For this review, take the finished solid that the model builds, in its own axes (mm). Face numbers are marked on the shaded views. Coordinates: 2 decimals unless noted, no trailing zeros. Order: outer loops, then holes, each group sorted by start corner. A loop starts at its lowest first (then second) coordinate and runs counter-clockwise, first axis right, second up. Notation, with made-up numbers: (61.25, 10.5) -> (91.25, 10.5) arc R22 cw to (91.25, 33.5) -> close; hole circle Ø5 at (20, -26). An arc over 180 degrees is marked (long way). Return JSON: item names as keys, results as strings. Group by question number.
Item 1: Take a section at B-B (z = -2.3). Write out the cut boundary in (x, y).
Item 2: Draft analysis for pull direction Z (two halves, no side actions). For the marked faces 1, 2 and 3, state which applies: +Z half, -Z half, draft (parallel to the pull), parting line (faces both ways), or undercut.
Item 3: Insertion check: pin 1 (0.5 mm diameter, centred on x = 4, y = 4.5, fed in from +Z); pin 2 (1.5 mm diameter, centred on x = 0.5, z = -2, fed in from +Y); pin 3 (0.5 mm diameter, centred on y = -0.5, z = -1.5, fed in from +X). Each pin has a flat end and moves straight along its axis. Give the tip position at first contact, or say it passes through.
Item 4: Take a section at A-A (y = 6.25). Write out the cut boundary in (x, z).
Item 5: Take a section at C-C (x = 4.45). Write out the cut boundary in (y, z), then the cut area to 3 significant figures.
Item 6: Take a section at D-D (y = 1.25). Write out the cut boundary in (x, z).
Item 7: For line 1 along X through (y, z) = (-1.25, -1.1); line 2 along Y through (x, z) = (3, -1.85); line 3 along Z through (x, y) = (1.5, 7), list the stretches that pass through material, from the lowest coordinate up.
```python
from build123d import *
from OCP.BRepFilletAPI import BRepFilletAPI_MakeChamfer

# Parameters (mm, degrees)
BOSS_EXTRUDE1_DEPTH         = 2.5
SKETCH2_W                   = 5.04
SKETCH2_H                   = 1.5
CUT_EXTRUDE1_DEPTH          = 0.5
SKETCH4_W                   = 0.04
SKETCH4_H                   = 1.8
CUT_EXTRUDE2_DEPTH          = 0.04
BOSS_EXTRUDE2_START         = -5.5
SKETCH3_W                   = 0.64
SKETCH3_H                   = 0.64
BOSS_EXTRUDE2_DEPTH         = 11.5
CHAMFER1_SIZE               = 0.2
CHAMFER1_SIZE2              = 0.140041508
LPATTERN1_COUNT             = 2
LPATTERN1_PITCH             = 2.54
CHAMFER1_OF_LPATTERN1_SIZE  = 0.2
CHAMFER1_OF_LPATTERN1_SIZE2 = 0.140041508


with BuildPart() as part:
    # Sketch1 → Boss-Extrude1 (new body)
    with BuildSketch(Plane(origin=(0, 0, 0), x_dir=(1, 0, 0), z_dir=(0, 1, 0))):
        Polygon((0, 2.15), (0.35, 2.5), (2.15, 2.5), (2.5, 2.15), (2.54, 2.15), (2.89, 2.5), (4.69, 2.5), (5.04, 2.15), (5.04, 0.35), (4.69, 0), (2.89, 0), (2.54, 0.35), (2.5, 0.35), (2.15, 0), (0.35, 0), (0, 0.35), align=None)
    extrude(amount=BOSS_EXTRUDE1_DEPTH)

    # Sketch2 → Cut-Extrude1 (cut)
    with BuildSketch(Plane.XZ):
        with Locations((2.52, -1.25)):
            Rectangle(SKETCH2_W, SKETCH2_H)
    extrude(amount=-CUT_EXTRUDE1_DEPTH, mode=Mode.SUBTRACT)

    # Sketch4 → Cut-Extrude2 (cut)
    with BuildSketch(Plane(origin=(0, 2.5, 0), x_dir=(1, 0, 0), z_dir=(0, 1, 0))):
        with Locations((5.06, 1.25)):
            Rectangle(SKETCH4_W, SKETCH4_H)
        with Locations((2.52, 1.25)):
            Rectangle(SKETCH4_W, SKETCH4_H)
        with Locations((7.6, 1.25)):
            Rectangle(SKETCH4_W, SKETCH4_H)
        with Locations((10.14, 1.25)):
            Rectangle(SKETCH4_W, SKETCH4_H)
        with Locations((12.68, 1.25)):
            Rectangle(SKETCH4_W, SKETCH4_H)
        with Locations((15.22, 1.25)):
            Rectangle(SKETCH4_W, SKETCH4_H)
        with Locations((17.76, 1.25)):
            Rectangle(SKETCH4_W, SKETCH4_H)
    extrude(amount=-CUT_EXTRUDE2_DEPTH, mode=Mode.SUBTRACT)

    # Sketch3 → Boss-Extrude2 (add)
    with BuildSketch(Plane(origin=(0, 2.5, 0), x_dir=(1, 0, 0), z_dir=(0, 1, 0)).offset(BOSS_EXTRUDE2_START)):
        with Locations((1.25, 1.25)):
            Rectangle(SKETCH3_W, SKETCH3_H)
    boss_extrude2 = extrude(amount=BOSS_EXTRUDE2_DEPTH)

    # Chamfer1: one chamfer whose edges measure the first distance from different faces: ONE call of the kernel's chamfer builder (chamfer() names one face for all edges)
    chamfer1_edges_1 = [part.edges().sort_by_distance(p)[0] for p in [
        (1.57, -3, -1.25),
    ]]
    chamfer1_side_1 = [part.faces().sort_by_distance(p)[0] for p in [
        (1.57, -1.25, -1.25),
    ]]
    chamfer1_edges_2 = [part.edges().sort_by_distance(p)[0] for p in [
        (1.25, -3, -0.93),
    ]]
    chamfer1_side_2 = [part.faces().sort_by_distance(p)[0] for p in [
        (1.25, -1.25, -0.93),
    ]]
    chamfer1_edges_3 = [part.edges().sort_by_distance(p)[0] for p in [
        (0.93, -3, -1.25),
    ]]
    chamfer1_side_3 = [part.faces().sort_by_distance(p)[0] for p in [
        (0.93, -1.25, -1.25),
    ]]
    chamfer1_edges_4 = [part.edges().sort_by_distance(p)[0] for p in [
        (1.25, -3, -1.57),
    ]]
    chamfer1_side_4 = [part.faces().sort_by_distance(p)[0] for p in [
        (1.25, -1.25, -1.57),
    ]]
    chamfer1_edges_5 = [part.edges().sort_by_distance(p)[0] for p in [
        (1.57, 8.5, -1.25),
    ]]
    chamfer1_side_5 = [part.faces().sort_by_distance(p)[0] for p in [
        (1.57, 5.5, -1.25),
    ]]
    chamfer1_edges_6 = [part.edges().sort_by_distance(p)[0] for p in [
        (1.25, 8.5, -1.57),
    ]]
    chamfer1_side_6 = [part.faces().sort_by_distance(p)[0] for p in [
        (1.25, 5.5, -1.57),
    ]]
    chamfer1_edges_7 = [part.edges().sort_by_distance(p)[0] for p in [
        (0.93, 8.5, -1.25),
    ]]
    chamfer1_side_7 = [part.faces().sort_by_distance(p)[0] for p in [
        (0.93, 5.5, -1.25),
    ]]
    chamfer1_edges_8 = [part.edges().sort_by_distance(p)[0] for p in [
        (1.25, 8.5, -0.93),
    ]]
    chamfer1_side_8 = [part.faces().sort_by_distance(p)[0] for p in [
        (1.25, 5.5, -0.93),
    ]]
    chamfer1 = BRepFilletAPI_MakeChamfer(part.part.solid().wrapped)
    for e in chamfer1_edges_1:
        chamfer1.Add(CHAMFER1_SIZE, CHAMFER1_SIZE2, e.wrapped, chamfer1_side_1[0].wrapped)  # the first distance lies on this face
    for e in chamfer1_edges_2:
        chamfer1.Add(CHAMFER1_SIZE, CHAMFER1_SIZE2, e.wrapped, chamfer1_side_2[0].wrapped)  # the first distance lies on this face
    for e in chamfer1_edges_3:
        chamfer1.Add(CHAMFER1_SIZE, CHAMFER1_SIZE2, e.wrapped, chamfer1_side_3[0].wrapped)  # the first distance lies on this face
    for e in chamfer1_edges_4:
        chamfer1.Add(CHAMFER1_SIZE, CHAMFER1_SIZE2, e.wrapped, chamfer1_side_4[0].wrapped)  # the first distance lies on this face
    for e in chamfer1_edges_5:
        chamfer1.Add(CHAMFER1_SIZE, CHAMFER1_SIZE2, e.wrapped, chamfer1_side_5[0].wrapped)  # the first distance lies on this face
    for e in chamfer1_edges_6:
        chamfer1.Add(CHAMFER1_SIZE, CHAMFER1_SIZE2, e.wrapped, chamfer1_side_6[0].wrapped)  # the first distance lies on this face
    for e in chamfer1_edges_7:
        chamfer1.Add(CHAMFER1_SIZE, CHAMFER1_SIZE2, e.wrapped, chamfer1_side_7[0].wrapped)  # the first distance lies on this face
    for e in chamfer1_edges_8:
        chamfer1.Add(CHAMFER1_SIZE, CHAMFER1_SIZE2, e.wrapped, chamfer1_side_8[0].wrapped)  # the first distance lies on this face
    add(Compound.cast(chamfer1.Shape()), mode=Mode.REPLACE)

    # LPattern1: Boss-Extrude2 ×2
    with Locations(*[(i * LPATTERN1_PITCH, 0, 0) for i in range(1, LPATTERN1_COUNT)]):
        add(boss_extrude2)

    # Chamfer1 of LPattern1: one chamfer whose edges measure the first distance from different faces: ONE call of the kernel's chamfer builder (chamfer() names one face for all edges)
    chamfer1_of_lpattern1_edges_1 = [part.edges().sort_by_distance(p)[0] for p in [
        (4.11, -3, -1.25),
    ]]
    chamfer1_of_lpattern1_side_1 = [part.faces().sort_by_distance(p)[0] for p in [
        (4.11, -1.25, -1.25),
    ]]
    chamfer1_of_lpattern1_edges_2 = [part.edges().sort_by_distance(p)[0] for p in [
        (3.79, -3, -0.93),
    ]]
    chamfer1_of_lpattern1_side_2 = [part.faces().sort_by_distance(p)[0] for p in [
        (3.79, -1.25, -0.93),
    ]]
    chamfer1_of_lpattern1_edges_3 = [part.edges().sort_by_distance(p)[0] for p in [
        (3.47, -3, -1.25),
    ]]
    chamfer1_of_lpattern1_side_3 = [part.faces().sort_by_distance(p)[0] for p in [
        (3.47, -1.25, -1.25),
    ]]
    chamfer1_of_lpattern1_edges_4 = [part.edges().sort_by_distance(p)[0] for p in [
        (3.79, -3, -1.57),
    ]]
    chamfer1_of_lpattern1_side_4 = [part.faces().sort_by_distance(p)[0] for p in [
        (3.79, -1.25, -1.57),
    ]]
    chamfer1_of_lpattern1_edges_5 = [part.edges().sort_by_distance(p)[0] for p in [
        (4.11, 8.5, -1.25),
    ]]
    chamfer1_of_lpattern1_side_5 = [part.faces().sort_by_distance(p)[0] for p in [
        (4.11, 5.5, -1.25),
    ]]
    chamfer1_of_lpattern1_edges_6 = [part.edges().sort_by_distance(p)[0] for p in [
        (3.79, 8.5, -1.57),
    ]]
    chamfer1_of_lpattern1_side_6 = [part.faces().sort_by_distance(p)[0] for p in [
        (3.79, 5.5, -1.57),
    ]]
    chamfer1_of_lpattern1_edges_7 = [part.edges().sort_by_distance(p)[0] for p in [
        (3.47, 8.5, -1.25),
    ]]
    chamfer1_of_lpattern1_side_7 = [part.faces().sort_by_distance(p)[0] for p in [
        (3.47, 5.5, -1.25),
    ]]
    chamfer1_of_lpattern1_edges_8 = [part.edges().sort_by_distance(p)[0] for p in [
        (3.79, 8.5, -0.93),
    ]]
    chamfer1_of_lpattern1_side_8 = [part.faces().sort_by_distance(p)[0] for p in [
        (3.79, 5.5, -0.93),
    ]]
    chamfer1_of_lpattern1 = BRepFilletAPI_MakeChamfer(part.part.solid().wrapped)
    for e in chamfer1_of_lpattern1_edges_1:
        chamfer1_of_lpattern1.Add(CHAMFER1_OF_LPATTERN1_SIZE, CHAMFER1_OF_LPATTERN1_SIZE2, e.wrapped, chamfer1_of_lpattern1_side_1[0].wrapped)  # the first distance lies on this face
    for e in chamfer1_of_lpattern1_edges_2:
        chamfer1_of_lpattern1.Add(CHAMFER1_OF_LPATTERN1_SIZE, CHAMFER1_OF_LPATTERN1_SIZE2, e.wrapped, chamfer1_of_lpattern1_side_2[0].wrapped)  # the first distance lies on this face
    for e in chamfer1_of_lpattern1_edges_3:
        chamfer1_of_lpattern1.Add(CHAMFER1_OF_LPATTERN1_SIZE, CHAMFER1_OF_LPATTERN1_SIZE2, e.wrapped, chamfer1_of_lpattern1_side_3[0].wrapped)  # the first distance lies on this face
    for e in chamfer1_of_lpattern1_edges_4:
        chamfer1_of_lpattern1.Add(CHAMFER1_OF_LPATTERN1_SIZE, CHAMFER1_OF_LPATTERN1_SIZE2, e.wrapped, chamfer1_of_lpattern1_side_4[0].wrapped)  # the first distance lies on this face
    for e in chamfer1_of_lpattern1_edges_5:
        chamfer1_of_lpattern1.Add(CHAMFER1_OF_LPATTERN1_SIZE, CHAMFER1_OF_LPATTERN1_SIZE2, e.wrapped, chamfer1_of_lpattern1_side_5[0].wrapped)  # the first distance lies on this face
    for e in chamfer1_of_lpattern1_edges_6:
        chamfer1_of_lpattern1.Add(CHAMFER1_OF_LPATTERN1_SIZE, CHAMFER1_OF_LPATTERN1_SIZE2, e.wrapped, chamfer1_of_lpattern1_side_6[0].wrapped)  # the first distance lies on this face
    for e in chamfer1_of_lpattern1_edges_7:
        chamfer1_of_lpattern1.Add(CHAMFER1_OF_LPATTERN1_SIZE, CHAMFER1_OF_LPATTERN1_SIZE2, e.wrapped, chamfer1_of_lpattern1_side_7[0].wrapped)  # the first distance lies on this face
    for e in chamfer1_of_lpattern1_edges_8:
        chamfer1_of_lpattern1.Add(CHAMFER1_OF_LPATTERN1_SIZE, CHAMFER1_OF_LPATTERN1_SIZE2, e.wrapped, chamfer1_of_lpattern1_side_8[0].wrapped)  # the first distance lies on this face
    add(Compound.cast(chamfer1_of_lpattern1.Shape()), mode=Mode.REPLACE)


solid = part.part
```
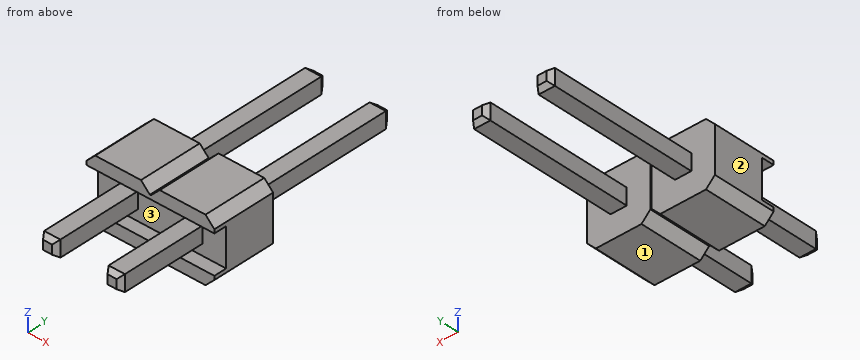
Findings below:
{
 "1": {"outline": "(0.15, 0) -> (2.35, 0) -> (2.35, 2.5) -> (0.15, 2.5) -> close; (2.69, 0) -> (4.89, 0) -> (4.89, 2.5) -> (2.69, 2.5) -> close"},
 "2": {"face 1": "-Z half", "face 2": "draft", "face 3": "undercut"},
 "3": {"pin 1": "stops at z = -0.93", "pin 2": "stops at y = 8.44", "pin 3": "stops at x = 4.11"},
 "4": {"outline": "(0.93, -1.57) -> (1.57, -1.57) -> (1.57, -0.93) -> (0.93, -0.93) -> close; (3.47, -1.57) -> (4.11, -1.57) -> (4.11, -0.93) -> (3.47, -0.93) -> close"},
 "5": {"outline": "(0, -2.5) -> (2.5, -2.5) -> (2.5, 0) -> (0, 0) -> (0, -0.5) -> (0.5, -0.5) -> (0.5, -2) -> (0, -2) -> close", "area": "5.50 mm2"},
 "6": {"outline": "(0, -2.15) -> (0.35, -2.5) -> (2.15, -2.5) -> (2.5, -2.15) -> (2.54, -2.15) -> (2.89, -2.5) -> (4.69, -2.5) -> (5.04, -2.15) -> (5.04, -0.35) -> (4.69, 0) -> (2.89, 0) -> (2.54, -0.35) -> (2.5, -0.35) -> (2.15, 0) -> (0.35, 0) -> (0, -0.35) -> close"},
 "7": {"line 1": "x = 0.93 to 1.57, 3.47 to 4.11", "line 2": "y = 0.5 to 2.5", "line 3": "z = -1.57 to -0.93"}
}
